Check sheet for the modelled part. Datum: model origin and axes. Units: mm. Face numbers are marked on the shaded views. Give positions to 0.01 mm unless a question says otherwise; leave off trailing zeros. Write each loop counter-clockwise with the first axis right and the second up, starting at its lowest first coordinate (ties: lowest second). Pieces come first, ordered by that corner, then holes. Notation, with made-up numbers: M -17.5,-38 L 12.5,-38 A24 cw 12.5,-14 Z; hole C -11,58 d2. An arc over 180 degrees is marked long. Write item = value, one per line. Start each with the question number.
1) Cross-section at C-C, the plane x = 90. Record the cut outline in (y, z).
2) Go/stop test with flat-tipped pins: pin 1 (10 mm diameter, centred on x = 34.5, z = 39, fed in from -Y); pin 2 (3 mm diameter, centred on y = -15, z = 34, fed in from -X); pin 3 (2.5 mm diameter, centred on x = 28, y = -15, fed in from +Z). Record where each tip stops, or that it passes through.
3) Cross-section at A-A, the plane x = 29. Record the cut outline in (y, z).
4) Scan lines: line 1 along X through (y, z) = (-12.75, 30); line 2 along Z through (x, y) = (60, -14); line 3 along Y through (x, z) = (29, 43). Record each from-to range of solid material in increasing order. Write a range as [from, to].
5) Mould release check, pull along X, two halves, no side actions. Record for the marked faces 1, 2, 3 and 4: released by +X, released by -X, zero draft, split by the parting line, or undercut.
6) Cross-section at B-B, the plane z = 41.5. Record the cut outline in (x, y), plus the area to 3 significant figures.
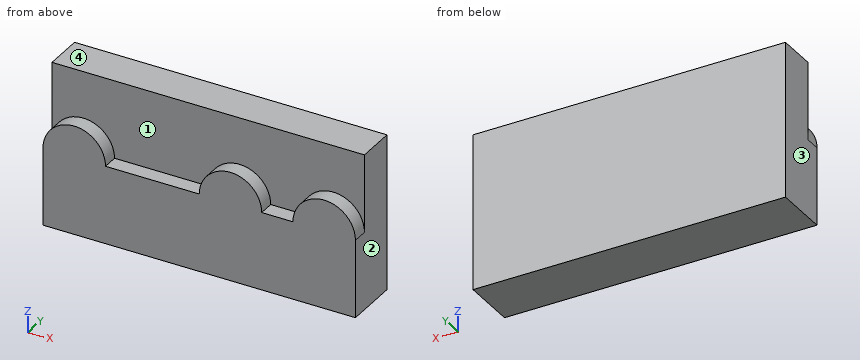
```python
from build123d import *

# Parameters (mm, degrees)
F0_W     = 100
F0_H     = 50
F1_DEPTH = 12.5
F3_DEPTH = 5


with BuildPart() as f1:
    # F0 (on Front) → F1 (new body)
    with BuildSketch(Plane.XZ):
        with Locations((50, 25)):
            Rectangle(F0_W, F0_H)
    extrude(amount=F1_DEPTH)

    # F2 (on face) → F3 (join)
    with BuildSketch(Plane.XZ.offset(12.5)):
        Polygon((20, 25), (0, 25), (0, 0), (100, 0), (100, 25), (80, 25), (70, 25), (50, 25), align=None)
        with BuildLine():
            ThreePointArc((20, 25), (10, 35), (0, 25))
            Line((0, 25), (20, 25))
        make_face()
        with BuildLine():
            ThreePointArc((70, 25), (60, 35), (50, 25))
            Line((50, 25), (70, 25))
        make_face()
        with BuildLine():
            Line((80, 25), (100, 25))
            ThreePointArc((100, 25), (90, 35), (80, 25))
        make_face()
    extrude(amount=F3_DEPTH)


solid = f1.part
```
Reply:
q1.outline = M -17.5,0 L 0,0 L 0,50 L -12.5,50 L -12.5,35 L -17.5,35 Z
q2.pin_1 = -12.5
q2.pin_2 = 3.39
q2.pin_3 = 25
q3.outline = M -17.5,0 L 0,0 L 0,50 L -12.5,50 L -12.5,25 L -17.5,25 Z
q4.line_1 = [1.34, 18.66], [51.34, 68.66], [81.34, 98.66]
q4.line_2 = [0, 35]
q4.line_3 = [-12.5, 0]
q5.face_1 = undercut
q5.face_2 = released by +X
q5.face_3 = released by -X
q5.face_4 = zero draft
q6.outline = M 0,-12.5 L 100,-12.5 L 100,0 L 0,0 Z
q6.area = 1,250 mm2
